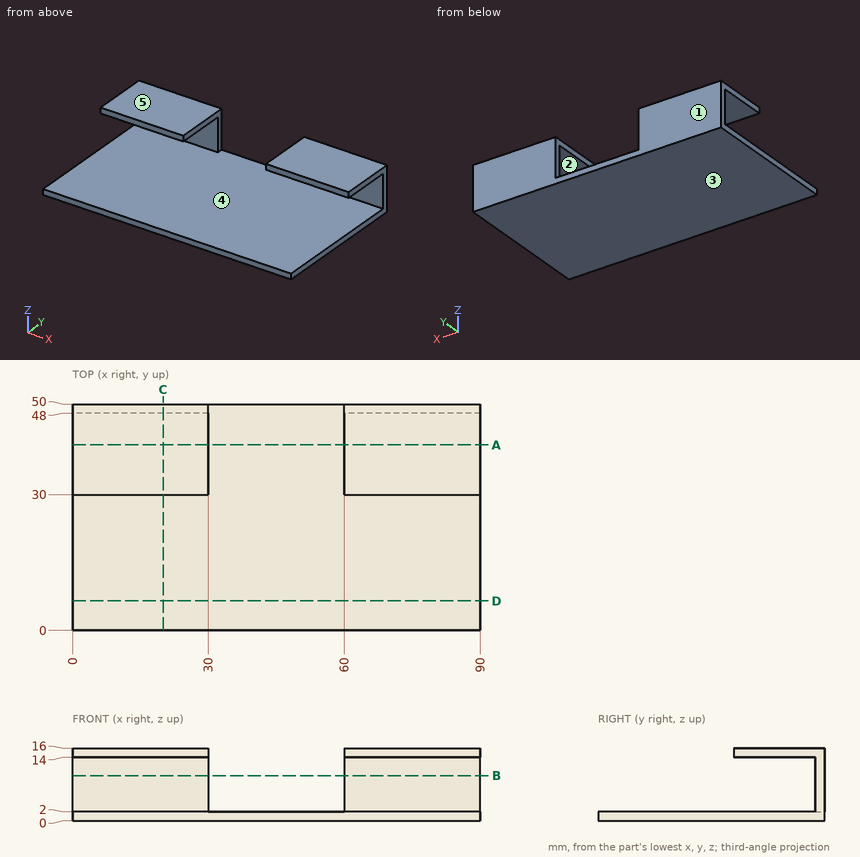
The figure shows three views and two pictorial views of one solid part (mm, origin at its lowest corner). Answer the questions. A direction names the side the tool comes from. Coordinates: 2 decimals unless noted, no trailing zeros. Loops run counter-clockwise (first coordinate to the right, second up) from the corner with the lowest first, then second, coordinate; pieces in that order, holes last. Notation, with made-up numbers: (35.5, -3) -> (50.5, -3) arc R30 cw to (50.5, 30) -> close; hole circle Ø2 at (34, -27.5). An arc over 180 degrees is marked (long way). Return JSON: item names as keys, results as strings. Group by question number.
(1) Given pin 1 Ø2 at (x, z) = (71, 15) entering from -Y; pin 2 Ø4 at (y, z) = (44.5, 10) entering from -X; pin 3 Ø2 at (x, z) = (74, 8) entering from -Y; pin 4 Ø8 at (x, y) = (62, 16.5) entering from +Z, each flat-ended and moving along its own axis, determine where each tip first touches the part or whether it passes through.
(2) A cutting plane is placed at B-B on z = 10. Write down the section's boundary in (x, y).
(3) A cutting plane is placed at D-D on y = 6.5. Write down the section's boundary in (x, z), and give its area (3 significant figures).
(4) A cutting plane is placed at A-A on y = 41. Write down the section's boundary in (x, z).
(5) Which of the six approach directions +Z, -Z, +X, -X, +Y, -Y give full straight-line access (tool end or side, diameter ignored) to the marked faces 1 and 2?
(6) A cutting plane is placed at C-C on x = 20. Write down the section's boundary in (y, z).
(7) Determine the mould class of the marked faces 3, 4 and 5 for opening direction Z: released by +Z, released by -Z, zero draft, split by the parting line, or undercut.
(8) Find the intervals of material crossed by probe 1 along Z at (x, y) = (19.5, 35); probe 2 along Y at (x, z) = (75, 11.25); probe 3 along Z at (x, y) = (74, 13.5), in increasing order. Write a range as from..to.
The answers:
{
 "1": {"pin 1": "stops at y = 30", "pin 2": "passes through", "pin 3": "stops at y = 48", "pin 4": "stops at z = 2"},
 "2": {"outline": "(0, 48) -> (30, 48) -> (30, 50) -> (0, 50) -> close; (60, 48) -> (90, 48) -> (90, 50) -> (60, 50) -> close"},
 "3": {"outline": "(0, 0) -> (90, 0) -> (90, 2) -> (0, 2) -> close", "area": "180 mm^2"},
 "4": {"outline": "(0, 0) -> (90, 0) -> (90, 2) -> (0, 2) -> close; (0, 14) -> (30, 14) -> (30, 16) -> (0, 16) -> close; (60, 14) -> (90, 14) -> (90, 16) -> (60, 16) -> close"},
 "5": {"face 1": "+Z, -Z, +X, -X, +Y", "face 2": "+X, -X, -Y"},
 "6": {"outline": "(0, 0) -> (50, 0) -> (50, 16) -> (30, 16) -> (30, 14) -> (48, 14) -> (48, 2) -> (0, 2) -> close"},
 "7": {"face 3": "released by -Z", "face 4": "undercut", "face 5": "released by +Z"},
 "8": {"probe 1": "z = 0..2, 14..16", "probe 2": "y = 48..50", "probe 3": "z = 0..2"}
}
